Autodesk Inventor part; units mm, degrees
ref_plane "YZ Plane" through (0, 0, 0) normal (1, 0, 0) x (0, 1, 0)
ref_plane "XZ Plane" through (0, 0, 0) normal (0, 1, 0) x (-1, 0, 0)
ref_plane "XY Plane" through (0, 0, 0) normal (0, 0, 1) x (1, 0, 0)
ref_plane "Work Plane3" through (0, 6, 0) normal (0, 1, 0) x (1, 0, 0)
sketch "Sketch2" plane through (0, 6, 0) normal (0, 1, 0) x (1, 0, 0)
  line L0 (0, 0) -> (0, 22.5)
  line L1 (0, 45) -> (0, 0)
  line L2 (0, 22.5) -> (22.5, 22.5)
  circle A0 centre (22.5, 22.5) radius 22.5
  dimension "d5" = 22.5
  dimension "d6" = 22.5
  dimension "d7" = 45
extrude "Extrusion2" add sketch "Sketch2" along normal blind 33.5
ref_plane "Work Plane2" through (0, 0, 0) normal (0, -1, 0) x (1, 0, 0)
sketch "Sketch3" plane through (0, 0, 0) normal (0, -1, 0) x (1, 0, 0)
  line L0 (0, -45) -> (0, 0)
  line L1 (0, 0) -> (0, -22.5)
  circle A0 centre (22.5, -22.5) radius 18.25
  dimension "d12" = 36.5
extrude "Extrusion3" cut sketch "Sketch3" against normal blind 65
sketch "Sketch4" plane through (22.5, 39.5, -22.5) normal (0, 1, 0) x (1, 0, 0)
  circle A0 centre (0, 0) radius 6.75
  point P0 (-22.5, -22.5)
  dimension "d15" = 13.5
extrude "Extrusion4" cut sketch "Sketch4" against normal blind 4.5
ref_plane "Work Plane1" through (0, 0, 0) normal (0, -1, 0) x (1, 0, 0)
sketch "Sketch5" plane through (0, 0, 0) normal (0, -1, 0) x (1, 0, 0)
  line L0 (0, -45) -> (0, 0)
  line L1 (0, 0) -> (22.5, 0)
  line L2 (0, 0) -> (45, 0)
sketch "Sketch6" plane through (22.5, 39.5, -22.5) normal (0, 1, 0) x (1, 0, 0)
  point P0 (-22.5, -22.5)
sketch "Sketch7" plane through (22.5, 39.5, -22.5) normal (0, 1, 0) x (1, 0, 0)
  circle A0 centre (0, 0) radius 18.25
  circle A1 centre (0, 0) radius 18.25
  point P0 (-22.5, -22.5)
extrude "Extrusion5" add sketch "Sketch7" against normal blind 3.5
sketch "Sketch8" plane through (22.5, 39.5, -22.5) normal (0, 1, 0) x (1, 0, 0)
  circle A0 centre (0, 0) radius 6.75
  point P0 (-22.5, -22.5)
  dimension "d20" = 13.5
extrude "Extrusion6" cut sketch "Sketch8" against normal blind 3.5
sketch "Sketch9" plane through (22.5, 6, -22.5) normal (0, -1, 0) x (1, 0, 0)
  point P0 (-22.5, 22.5)
sketch "Sketch10" plane through (22.5, 39.5, -22.5) normal (0, 1, 0) x (1, 0, 0)
  point P0 (-22.5, -22.5)
sketch "Sketch11" plane through (22.5, 6, -22.5) normal (0, -1, 0) x (1, 0, 0)
  circle A0 centre (0, 0) radius 22.5
  line L0 (0, 29) -> (32.5, 29)
  line L1 (32.5, 29) -> (32.5, -29)
  line L2 (32.5, -29) -> (-32.5, -29)
  line L3 (0, 29) -> (-32.5, 29)
  point P0 (-22.5, 22.5)
  dimension "d25" = 58
  dimension "d26" = 65
  dimension "d27" = 32.5
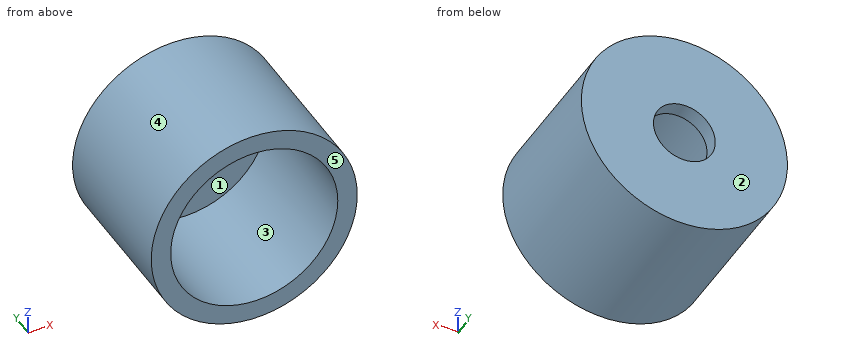
Geometry check sheet. Reference: the model listing, model coordinates, mm. Face numbers are marked on the shaded views. A direction names the side the tool comes from. Round coordinates to 2 decimals unless told otherwise and drop trailing zeros. Order: outer loops, then holes, each group sorted by start corner. A loop starts at its lowest first (then second) coordinate and runs counter-clockwise, first axis right, second up. Notation, with made-up numbers: (-34.5, -24) - (-2.5, -24) arc R27 cw to (-2.5, 7) - close; hole circle Ø11 at (38, 9). An arc over 180 degrees is marked (long way). Use a Markdown table: item, result. Add a question column.
(1) Material ranges on line 1 along Z through (x, y) = (22, 18); line 2 along X through (y, z) = (21.5, -22); line 3 along X through (y, z) = (37, -22), recorded low to high. Write a range as [from, to].
(2) Sectioned sample at A-A, the plane x = 22.5. Enter the section's corners in (y, z).
(3) Release check for a two-part mould opening along X. For the marked faces 3, 4 and 5 record: pulls with the +X half, pulls with the -X half, needs draft (parallel to the pull), parting line crosses it, or undercut.
(4) Depth check by flat-ended pin: pin 1 (8 mm diameter, centred on x = 37.5, y = 27.5, fed in from +Z); pin 2 (12 mm diameter, centred on x = 18, y = 20, fed in from -Z); pin 3 (6 mm diameter, centred on y = 34.5, z = -13, fed in from +X). Enter the tip coordinate at first touch or a pass-through.
(5) Sectioned sample at B-B, the plane z = -22.5. Enter the section's corners in (x, y), and give its area (3 significant figures).
(6) Sectioned sample at C-C, the plane y = 21.5. Enter the section's corners in (x, z), and give its area (3 significant figures).
(7) Tool access check on the marked faces 1 and 2. Record the directions out of +Z, -Z, +X, -X, +Y, -Y that give a thin tool (end or side, any length) a straight path to the whole face; none if there is none.
(8) Sectioned sample at D-D, the plane x = 15. Enter the section's corners in (y, z), and give its area (3 significant figures).
Answers below:
| question | item | result |
|---|---|---|
| 1 | line 1 | [-44.99, -40.74], [-4.26, -0.01] |
| 1 | line 2 | [0.01, 4.26], [40.74, 44.99] |
| 1 | line 3 | [0.01, 15.77], [29.23, 44.99] |
| 2 | outline | (6, -45) - (39.5, -45) - (39.5, -29.25) - (36, -29.25) - (36, -40.75) - (6, -40.75) - close; (6, -4.25) - (36, -4.25) - (36, -15.75) - (39.5, -15.75) - (39.5, 0) - (6, 0) - close |
| 3 | face 3 | undercut |
| 3 | face 4 | parting line crosses it |
| 3 | face 5 | needs draft |
| 4 | pin 1 | z = -2.87 |
| 4 | pin 2 | z = -45 |
| 4 | pin 3 | x = 44.04 |
| 5 | outline | (0, 6) - (4.25, 6) - (4.25, 36) - (15.75, 36) - (15.75, 39.5) - (0, 39.5) - close; (29.25, 36) - (40.75, 36) - (40.75, 6) - (45, 6) - (45, 39.5) - (29.25, 39.5) - close |
| 5 | area | 365 mm² |
| 6 | outline | circle Ø45 at (22.5, -22.5); hole circle Ø36.5 at (22.5, -22.5) |
| 6 | area | 544 mm² |
| 7 | face 1 | -Y |
| 7 | face 2 | +Z, -Z, +X, -X, +Y |
| 8 | outline | (6, -43.71) - (39.5, -43.71) - (39.5, -1.29) - (6, -1.29) - (6, -5.86) - (36, -5.86) - (36, -39.14) - (6, -39.14) - close |
| 8 | area | 423 mm² |
